Work out the finished part from the listing and answer in its coordinate system (mm). A direction names the side the tool comes from. Give positions to 0.01 mm unless a question says otherwise; leave off trailing zeros. Loops run counter-clockwise (first coordinate to the right, second up) from the corner with the lowest first, then second, coordinate; pieces in that order, holes last. Notation, with made-up numbers: M 11,22 L 48,22 A33 ccw 48,60 Z; hole C 61.5,-23 d1. An arc over 180 degrees is marked long. Answer as a JSON object with one key per item and string values. Group by question number.
```python
from build123d import *

# Parameters (mm, degrees)
SKETCH_1_W          = 35
SKETCH_1_H          = 35
EXTRUDE_1_DEPTH     = 5.2
SKETCH_2_R          = 18
EXTRUDE_2_DEPTH     = 32.8
SKETCH_3_R          = 11
EXTRUDE_3_DEPTH     = 2
SKETCH_4_R          = 4
EXTRUDE_4_DEPTH     = 18
SKETCH_5_W          = 10.54681648
SKETCH_5_H          = 7.766292135
CUT_EXTRUDE_1_DEPTH = 15
CHAMFER_1_SIZE      = 2
SKETCH_6_R          = 1.5
CUT_EXTRUDE_2_DEPTH = 6


with BuildPart() as part:
    # 草图1 → 凸台-拉伸1 (new body)
    with BuildSketch(Plane(origin=(0, 0, 0), x_dir=(1, 0, 0), z_dir=(0, 1, 0))):
        Rectangle(SKETCH_1_W, SKETCH_1_H)
    extrude(amount=EXTRUDE_1_DEPTH)

    # 草图2 → 凸台-拉伸2 (add)
    with BuildSketch(Plane(origin=(0, 5.2, 0), x_dir=(1, 0, 0), z_dir=(0, 1, 0))):
        with Locations(Location((0, 0, 0), (0, 0, 76.463797263))):
            Circle(SKETCH_2_R)
    extrude(amount=EXTRUDE_2_DEPTH)

    # 草图3 → 凸台-拉伸3 (add)
    with BuildSketch(Plane(origin=(0, 38, 0), x_dir=(1, 0, 0), z_dir=(0, 1, 0))):
        with Locations(Location((0, 0, 0), (0, 0, 270))):
            Circle(SKETCH_3_R)
    extrude(amount=EXTRUDE_3_DEPTH)

    # 草图4 → 凸台-拉伸4 (add)
    with BuildSketch(Plane(origin=(0, 40, 0), x_dir=(1, 0, 0), z_dir=(0, 1, 0))):
        with Locations(Location((0, 0, 0), (0, 0, 270))):
            Circle(SKETCH_4_R)
    extrude(amount=EXTRUDE_4_DEPTH)

    # 草图5 → 切除-拉伸1 (cut)
    with BuildSketch(Plane(origin=(0, 58, 0), x_dir=(1, 0, 0), z_dir=(0, 1, 0))):
        with Locations((0, 6.883146068)):
            Rectangle(SKETCH_5_W, SKETCH_5_H)
    extrude(amount=-CUT_EXTRUDE_1_DEPTH, mode=Mode.SUBTRACT)

    # 倒角1
    chamfer_1_edges = [part.edges().sort_by_distance(p)[0] for p in [
        (17.5, 2.6, 17.5),
        (-17.5, 2.6, 17.5),
        (-17.5, 2.6, -17.5),
        (17.5, 2.6, -17.5),
    ]]
    chamfer(chamfer_1_edges, length=CHAMFER_1_SIZE)

    # 草图6 → 切除-拉伸2 (cut)
    with BuildSketch(Plane(origin=(0, 38, 0), x_dir=(1, 0, 0), z_dir=(0, 1, 0))):
        with Locations(Location((0, 14, 0), (0, 0, 270))):
            Circle(SKETCH_6_R)
        with Locations(Location((14, 0, 0), (0, 0, 270))):
            Circle(SKETCH_6_R)
        with Locations(Location((0, -14, 0), (0, 0, 270))):
            Circle(SKETCH_6_R)
        with Locations(Location((-14, 0, 0), (0, 0, 270))):
            Circle(SKETCH_6_R)
    extrude(amount=-CUT_EXTRUDE_2_DEPTH, mode=Mode.SUBTRACT)


solid = part.part
```
Item 1: A cutting plane is placed at C-C (y = 20). Determine the outline of the cut face in (x, z), and give its area (3 significant figures).
Item 2: A tool of negligible diameter and unlimited length cuts with its end or side. For faces 1 (the flat face through (-6.2, 38, -9.5)), 2 (the flat face through (0, 51, -3)), 3 (the flat face through (17.5, 3, 0)), 4 (the flat face through (0, 3, -17.5)), 5 (the flat face through (0, 3, 17.5)), from which of +Z, -Z, +X, -X, +Y, -Y can it reach the whole face along a straight path? Write none if from no direction.
Item 3: Find the intervals of material crossed by probe 1 along X at (y, z) = (35.05, 0); probe 2 along X at (y, z) = (34.6, 14); probe 3 along Y at (x, z) = (-12.5, -5), in increasing order. Write a range as [from, to].
Item 4: Given pin 1 Ø10.5 at (x, z) = (-13, -9.5) entering from +Y; pin 2 Ø0.6 at (x, z) = (18, 1.5) entering from -Y; pin 3 Ø4 at (x, y) = (1, 2.5) entering from +Z, each flat-ended and moving along its own axis, determine where each tip first touches the part or whether it passes through.
Item 5: A cutting plane is placed at B-B (x = 0). Determine the outline of the cut face in (y, z).
Item 6: A cutting plane is placed at A-A (z = 0). Determine the outline of the cut face in (x, y), and give its area (3 significant figures).
Item 7: A cutting plane is placed at D-D (x = -9.5). Determine the outline of the cut face in (y, z), and give its area (3 significant figures).
Item 8: For a pull along X with two mould halves and no side action, classify faces 6 (the flat face through (-14, 5.2, -14)), 7 (the flat face through (17, 3, -16)), 8 (the cylindrical face through (14.45, 35.04, 1.43)) as pulls with the +X half, pulls with the -X half, needs draft (parallel to the pull), parting line crosses it, or undercut.
The answers:
{
 "1": {"outline": "C 0,0 d36", "area": "1,020 mm^2"},
 "2": {"face 1": "+Y", "face 2": "-Z, +X, -X, +Y", "face 3": "+Z, -Z, +X, -Y", "face 4": "-Z, +X, -X, -Y", "face 5": "+Z, +X, -X, -Y"},
 "3": {"probe 1": "x = [-18, -15.5], [-12.5, 12.5], [15.5, 18]", "probe 2": "x = [-11.31, -1.5], [1.5, 11.31]", "probe 3": "y = [0, 38]"},
 "4": {"pin 1": "stops at y = 40", "pin 2": "stops at y = 5.2", "pin 3": "stops at z = 17.5"},
 "5": {"outline": "M 0,-17.5 L 5.2,-17.5 L 5.2,-18 L 38,-18 L 38,-15.5 L 32,-15.5 L 32,-12.5 L 38,-12.5 L 38,-11 L 40,-11 L 40,-4 L 43,-4 L 43,-3 L 58,-3 L 58,4 L 40,4 L 40,11 L 38,11 L 38,12.5 L 32,12.5 L 32,15.5 L 38,15.5 L 38,18 L 5.2,18 L 5.2,17.5 L 0,17.5 Z"},
 "6": {"outline": "M -18,5.2 L -17.5,5.2 L -17.5,0 L 17.5,0 L 17.5,5.2 L 18,5.2 L 18,38 L 15.5,38 L 15.5,32 L 12.5,32 L 12.5,38 L 11,38 L 11,40 L 4,40 L 4,58 L -4,58 L -4,40 L -11,40 L -11,38 L -12.5,38 L -12.5,32 L -15.5,32 L -15.5,38 L -18,38 Z", "area": "1,510 mm^2"},
 "7": {"outline": "M 0,-17.5 L 5.2,-17.5 L 5.2,-15.29 L 38,-15.29 L 38,-5.55 L 40,-5.55 L 40,5.55 L 38,5.55 L 38,15.29 L 5.2,15.29 L 5.2,17.5 L 0,17.5 Z", "area": "1,210 mm^2"},
 "8": {"face 6": "needs draft", "face 7": "pulls with the +X half", "face 8": "undercut"}
}
